from build123d import *

# Parameters (mm, degrees)
SKETCH1_R             = 100
SKETCH1_R_2           = 99.238
BOSS_EXTRUDE1_DEPTH   = 27.7
F_2_5MM_DOWEL_HOLE1_D = 2.5
F_2_5MM_DOWEL_HOLE2_D = 2.5
SKETCH6_W             = 7.35
SKETCH6_H             = 61
CUT_EXTRUDE1_DEPTH    = 145.108605038


with BuildPart() as part:
    # Sketch1 → Boss-Extrude1 (new body)
    with BuildSketch(Plane(origin=(0, 0, 0), x_dir=(0, 0, -1), z_dir=(1, 0, 0))):
        Circle(SKETCH1_R)
        Circle(SKETCH1_R_2, mode=Mode.SUBTRACT)
    extrude(amount=BOSS_EXTRUDE1_DEPTH)

    # Ø2.5mm Dowel Hole1 (through all)
    with Locations(Plane.XY.offset(100)):
        with Locations((24.525, 0), (3.175, 0)):
            Hole(F_2_5MM_DOWEL_HOLE1_D / 2)

    # Ø2.5mm Dowel Hole2 (through all)
    with Locations(Plane(origin=(0, 100, 0), x_dir=(1, 0, 0), z_dir=(0, 1, 0))):
        with Locations((24.525, 0), (3.175, 0)):
            Hole(F_2_5MM_DOWEL_HOLE2_D / 2)

    # Sketch6 → Cut-Extrude1 (cut, through all)
    with BuildSketch(Plane(origin=(0, 0, 0), x_dir=(-1, 0, 0), z_dir=(0, 0.7071067811865475, -0.7071067811865477))):
        with Locations((-24.525, 0)):
            Rectangle(SKETCH6_W, SKETCH6_H)
    extrude(amount=-CUT_EXTRUDE1_DEPTH, mode=Mode.SUBTRACT)


solid = part.part
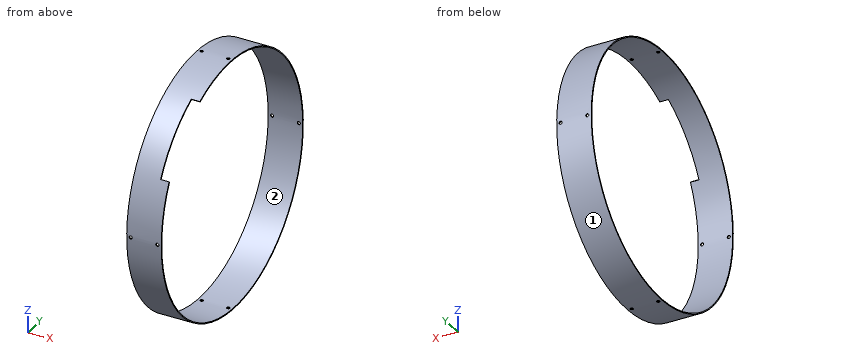
Here's how the part is built. I have some questions about the finished solid (model axes, mm). Face numbers are marked on the shaded views. Coordinates: 2 decimals unless noted, no trailing zeros. Order: outer loops, then holes, each group sorted by start corner. A loop starts at its lowest first (then second) coordinate and runs counter-clockwise, first axis right, second up.
Item 1: If we mould it in two halves opening along Z, with no side actions, what happens to the marked faces 1 and 2? For each: +Z half, -Z half, draft (parallel to the pull), parting line (faces both ways), or undercut.
Result sheet:
face 1: parting line
face 2: undercut
Item 2: If we section it at A-A on y = -64: List the corners of the cut face in (x, z) for me.
Result sheet:
outline: (0, -76.84) - (27.7, -76.84) - (27.7, -75.84) - (0, -75.84) - close; (0, 75.84) - (20.85, 75.84) - (20.85, 76.84) - (0, 76.84) - close
Item 3: If we section it at C-C on x = 8: List the corners of the cut face in (y, z) for me.
Result sheet:
outline: circle Ø200 at (0, 0); hole circle Ø198.48 at (0, 0)
Item 4: For P1, Ø1, axis at x = 23.5, z = 5.5, coming from the +Y side; P2, Ø1.5, axis at x = 3.175, z = 0, coming from the -Y side; P3, Ø12, axis at x = 14.5, z = 57.5, coming from the +Y side; P4, Ø13, axis at y = -70.5, z = 62.5, coming from the +X side, each with a flat end and sliding along its axis, tell me the tip position at first contact or that it passes through.
Result sheet:
P1: stops at y = 99.87
P2: passes through
P3: stops at y = 85.72
P4: stops at x = 20.85
Item 5: If we section it at B-B on z = 37: List the corners of the cut face in (x, y) for me.
Result sheet:
outline: (0, -92.9) - (27.7, -92.9) - (27.7, -92.08) - (0, -92.08) - close; (0, 92.08) - (27.7, 92.08) - (27.7, 92.9) - (0, 92.9) - close
Item 6: I need wall thicknesses on line 1 (Y direction, x = 9.25, z = 0); line 2 (X direction, y = 0, z = -99.5) (3 decimals); line 3 (Z direction, x = 5.25, y = -46.5). Which ranges of each line are inside material? Lowest first, please.
Result sheet:
line 1: y = -100 to -99.24, 99.24 to 100
line 2: x = 0 to 1.925, 4.425 to 23.275, 25.775 to 27.7
line 3: z = -88.53 to -87.67, 87.67 to 88.53
